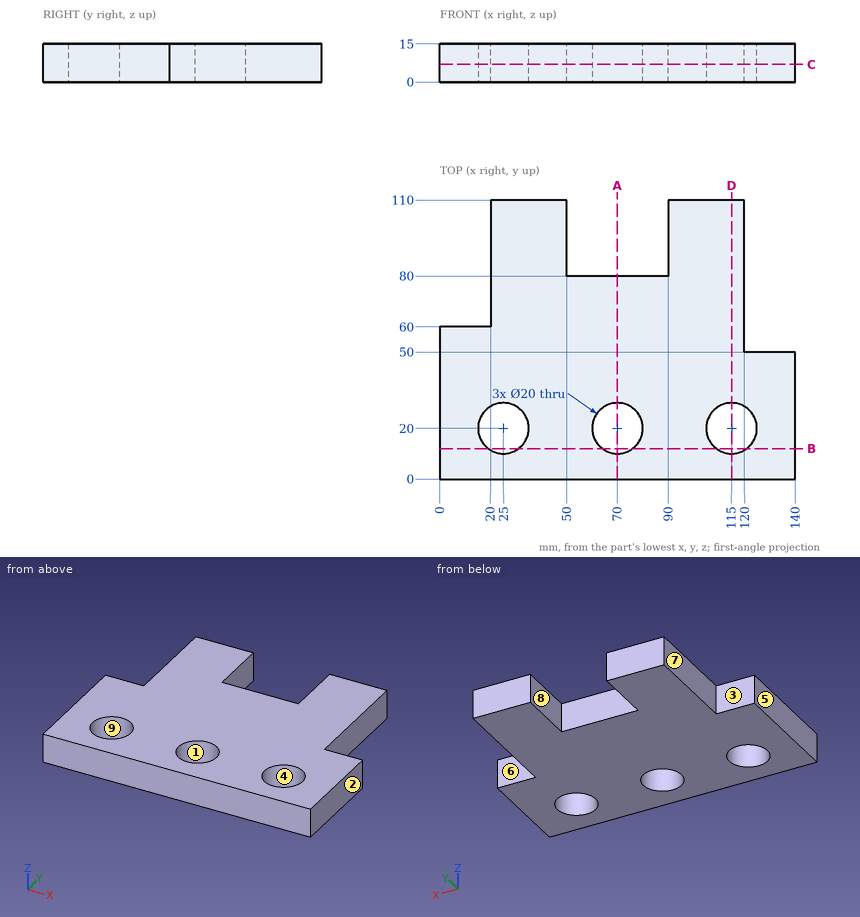
Answer from the drawing. Dimensions are ordinates in mm from the lowest x, y and z of the part. A direction names the side the tool comes from. Give positions to 0.01 mm unless a question says otherwise; leave off trailing zeros. Loops run counter-clockwise (first coordinate to the right, second up) from the corner with the lowest first, then second, coordinate; pieces in that order, holes last. Notation, with made-up numbers: (40.25, -8) - (78.25, -8) arc R5 cw to (78.25, -4) - close; hole circle Ø2 at (63.5, 1). An arc over 180 degrees is marked (long way). Answer as CSV lines item,"result". Start each with the question number.
Item 1: Each of these flat-tipped pins is pushed along its axis until it touches: pin 1 (6 mm diameter, centred on x = 73.5, z = 6, fed in from +Y); pin 2 (7.5 mm diameter, centred on x = 6.5, z = 4, fed in from +Y); pin 3 (7.5 mm diameter, centred on y = 79, z = 5.5, fed in from +X). Where does it stop, or does it pass through?
Item 2: The mould has two halves that part along Y. Classify the marked faces 1, 2, 3 and 4: +Y half, -Y half, draft (parallel to the pull), parting line (faces both ways), or undercut.
Item 3: Find the intervals of material crossed by line 1 (Y direction, x = 115, z = 11.25); line 2 (X direction, y = 100, z = 4.25); line 3 (Y direction, x = 70, z = 4.25), in increasing order. Write a range as from..to.
Item 4: A cutting plane is placed at C-C on z = 7. Determine the outline of the cut face in (x, y), then the cut area to 3 significant figures.
Item 5: For the marked faces 5, 6, 7, 8 and 9, determine the directions among +Z, -Z, +X, -X, +Y, -Y from which every point of the face is accessible in a straight line to the end or side of a thin tool.
Item 6: A cutting plane is placed at A-A on x = 70. Determine the outline of the cut face in (y, z).
Item 7: A cutting plane is placed at B-B on y = 12. Determine the outline of the cut face in (x, z), then the cut area to 3 significant figures.
Item 8: A cutting plane is placed at D-D on x = 115. Determine the outline of the cut face in (y, z).
Found:
1,pin 1,"stops at y = 80"
1,pin 2,"stops at y = 60"
1,pin 3,"stops at x = 120"
2,face 1,"undercut"
2,face 2,"draft"
2,face 3,"+Y half"
2,face 4,"undercut"
3,line 1,"y = 0..10, 30..110"
3,line 2,"x = 20..50, 90..120"
3,line 3,"y = 0..10, 30..80"
4,outline,"(0, 0) - (140, 0) - (140, 50) - (120, 50) - (120, 110) - (90, 110) - (90, 80) - (50, 80) - (50, 110) - (20, 110) - (20, 60) - (0, 60) - close; hole circle Ø20 at (25, 20); hole circle Ø20 at (70, 20); hole circle Ø20 at (115, 20)"
4,area,"11,100 mm^2"
5,face 5,"+Z, -Z, -X, +Y, -Y"
5,face 6,"+Z, -Z, +X, +Y"
5,face 7,"+Z, -Z, -X, +Y"
5,face 8,"+Z, -Z, +Y"
5,face 9,"+Z, -Z"
6,outline,"(0, 0) - (10, 0) - (10, 15) - (0, 15) - close; (30, 0) - (80, 0) - (80, 15) - (30, 15) - close"
7,outline,"(0, 0) - (19, 0) - (19, 15) - (0, 15) - close; (31, 0) - (64, 0) - (64, 15) - (31, 15) - close; (76, 0) - (109, 0) - (109, 15) - (76, 15) - close; (121, 0) - (140, 0) - (140, 15) - (121, 15) - close"
7,area,"1,560 mm^2"
8,outline,"(0, 0) - (10, 0) - (10, 15) - (0, 15) - close; (30, 0) - (110, 0) - (110, 15) - (30, 15) - close"
